Geometry check sheet. Reference: the model listing, model coordinates, mm. Round coordinates to 2 decimals unless told otherwise and drop trailing zeros. Write each loop counter-clockwise with the first axis right and the second up, starting at its lowest first coordinate (ties: lowest second). Pieces come first, ordered by that corner, then holes. Notation, with made-up numbers: M -21.5,-6.75 L 32.5,-6.75 A24 ccw 32.5,7.25 Z; hole C 59,44 d7. An arc over 180 degrees is marked long. Put each result on its own line as item: value. Start each with the question number.
(1) Section check A-A on x = 1.8. Record the cut outline in (y, z).
(2) Material ranges on probe 1 along Z at (x, y) = (3.4, 27.75); probe 2 along Z at (x, y) = (2.7, 28.5); probe 3 along Y at (x, z) = (1.5, 34), recorded low to high.
(3) Gauge pin test, flat ends, axial feed: pin 1 (1 mm diameter, centred on x = 2, y = 34, fed in from -Z); pin 2 (10.5 mm diameter, centred on y = 28.02, z = 66.04, fed in from +X). Record the tip position at first contact, or that the pin passes through.
(4) Section check C-C on z = -41. Record the cut outline in (x, y).
(5) Section check B-B on y = 41.25. Record the cut outline in (x, z).
Autodesk Inventor part; units mm, degrees
ref_plane "YZ Plane" through (0, 0, 0) normal (1, 0, 0) x (0, 1, 0)
ref_plane "XZ Plane" through (0, 0, 0) normal (0, 1, 0) x (-1, 0, 0)
ref_plane "XY Plane" through (0, 0, 0) normal (0, 0, 1) x (1, 0, 0)
sketch "Sketch1" plane through (0, 0, 0) normal (1, 0, 0) x (0, 1, 0)
  arc A0 (43.0231, 66.0406) -> (13.0231, 66.0406) centre (28.0231, 66.0406) ccw
  arc A1 (13.0231, -33.9594) -> (43.0231, -33.9594) centre (28.0231, -33.9594) ccw
  line L0 (13.0231, 66.0406) -> (13.0231, -33.9594)
  line L1 (43.0231, 66.0406) -> (43.0231, -33.9594)
  circle A2 centre (28.0231, 66.0406) radius 5
  circle A3 centre (28.0231, -33.9594) radius 2
  circle A4 centre (28.0231, 34.0406) radius 2
  circle A5 centre (28.0231, -13.9594) radius 2
  point P0 (0, 0)
  dimension "d6" = 15
  dimension "d18" = 100
  dimension "d40" = 10
  dimension "d50" = 0
  dimension "d51" = 0
  dimension "d52" = 20
  dimension "d53" = 32
  dimension "d54" = 4
  dimension "d66" = 4
extrude "Extrusion6" add sketch "Sketch1" along normal blind 4
hole "Hole4" at (4, 28.0231, 66.0406) direction (-1, 0, 0) diameter 11.6 depth 0.8 tip angle 118
sketch "Sketch6" plane through (4, 0, 0) normal (1, 0, 0) x (0, 0, -1)
  circle A0 centre (33.9594, 28.0231) radius 2
  line L0 (32.0767, 27.3481) -> (32.0767, 28.6981)
  line L1 (32.0767, 28.6981) -> (30.7767, 28.6981)
  line L2 (30.7767, 28.6981) -> (30.7767, 27.3481)
  line L3 (30.7767, 27.3481) -> (32.0767, 27.3481)
  point P0 (0, 0)
  dimension "d77" = 1.35
  dimension "d78" = 1.3
extrude "Extrusion7" cut sketch "Sketch6" against normal through all contours A0 L3 L2 L1
properties part number "BaseJoint"
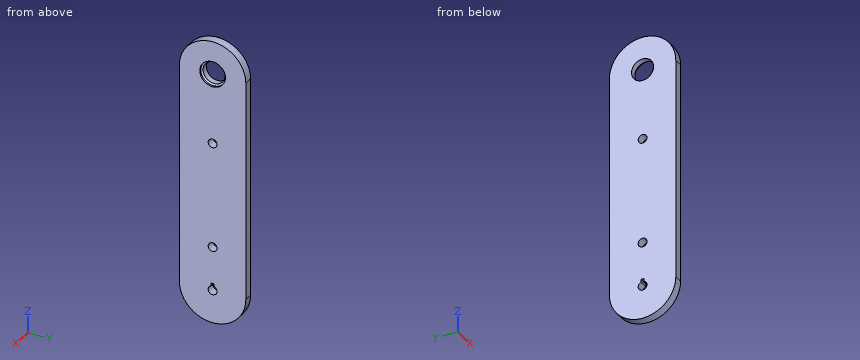
Answers follow:
1. outline: M 13.02,-33.96 A15 ccw 43.02,-33.96 L 43.02,66.04 A15 ccw 13.02,66.04 Z; hole C 28.02,66.04 d10; hole C 28.02,-13.96 d4; hole C 28.02,34.04 d4; hole M 27.35,-32.08 A2 ccw long 28.7,-32.08 L 28.7,-30.78 L 27.35,-30.78 Z
2. probe 1: z = -48.96 to -35.94, -30.78 to -15.94, -11.98 to 32.06, 36.02 to 60.25, 71.83 to 81.04
2. probe 2: z = -48.95 to -35.9, -30.78 to -15.9, -12.02 to 32.1, 35.98 to 61.06, 71.02 to 81.03
2. probe 3: y = 13.02 to 26.02, 30.02 to 43.02
3. pin 1: stops at z = -47.92
3. pin 2: stops at x = 2.87
4. outline: M 0,14.78 L 4,14.78 L 4,41.27 L 0,41.27 Z
5. outline: M 0,-41.03 L 4,-41.03 L 4,73.12 L 0,73.12 Z
